Design review of the part shown in the three views and the two pictorial views. Dimensions are in mm from the part's minimum x, y and z. A direction names the side the tool comes from. Coordinates: 2 decimals unless noted, no trailing zeros. Loops run counter-clockwise (first coordinate to the right, second up) from the corner with the lowest first, then second, coordinate; pieces in that order, holes last. Notation, with made-up numbers: (-29.75, -25) -> (20.25, -25) arc R7 ccw to (20.25, -19) -> close; hole circle Ø9 at (16.25, 14.25). An arc over 180 degrees is marked (long way). Answer in a Markdown table with one row per item.
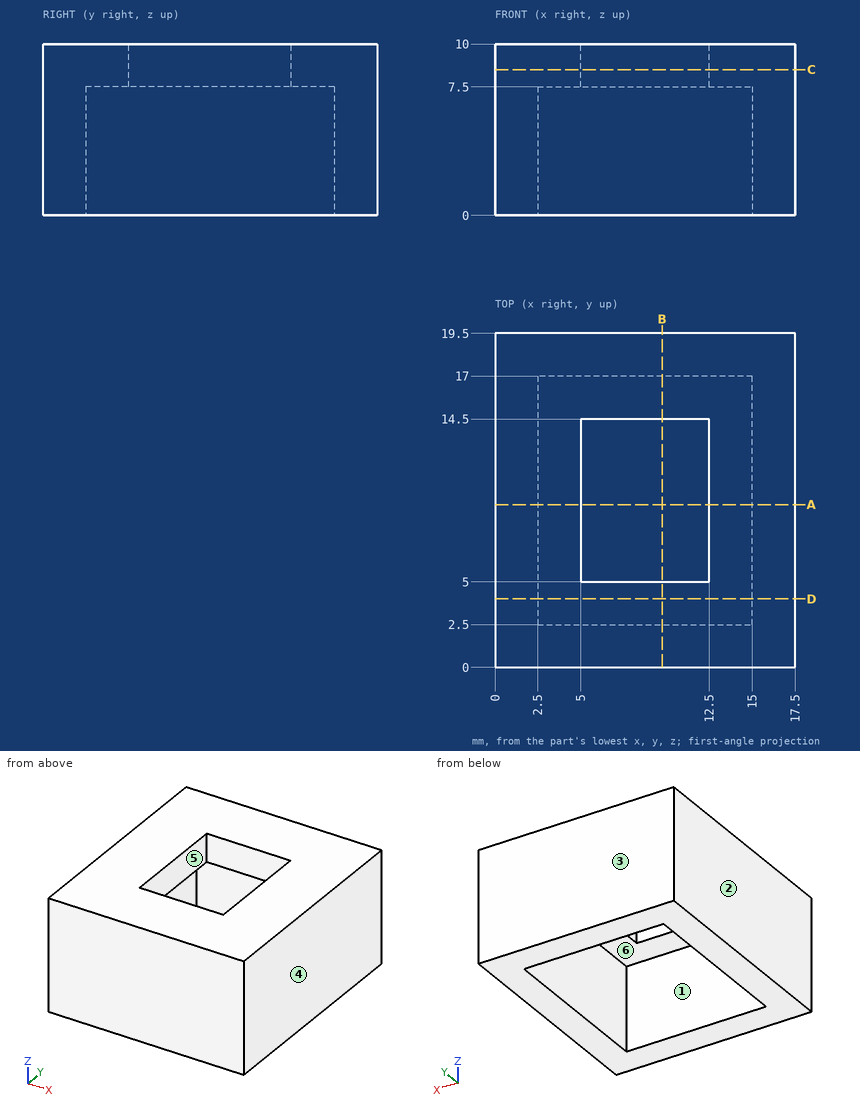
Item 1: Take a section at C-C, the plane z = 8.5. State the section outline as (x, y) points.
Worked answers:
| item | result |
|---|---|
| outline | (0, 0) -> (17.5, 0) -> (17.5, 19.5) -> (0, 19.5) -> close; hole (5, 5) -> (12.5, 5) -> (12.5, 14.5) -> (5, 14.5) -> close |
Item 2: For the marked faces 4, 5 and 6, list the 3-axis set-ups (+Z, -Z, +X, -X, +Y, -Y) from which the entire face can be reached by the end or side of a thin tool; tool diameter is ignored.
Worked answers:
| item | result |
|---|---|
| face 4 | +Z, -Z, +X, +Y, -Y |
| face 5 | +Z, -Z |
| face 6 | -Z |
Item 3: Take a section at A-A, the plane y = 9.5. State the section outline as (x, z) points.
Worked answers:
| item | result |
|---|---|
| outline | (0, 0) -> (2.5, 0) -> (2.5, 7.5) -> (5, 7.5) -> (5, 10) -> (0, 10) -> close; (12.5, 7.5) -> (15, 7.5) -> (15, 0) -> (17.5, 0) -> (17.5, 10) -> (12.5, 10) -> close |
Item 4: Insertion check: pin 1 (1.5 mm diameter, centred on y = 5.5, z = 8.5, fed in from -X); pin 2 (6 mm diameter, centred on x = 7, y = 11.5, fed in from -Z). Each pin has a flat end and moves straight along its axis. Give the tip position at first contact, or say it passes through.
Worked answers:
| item | result |
|---|---|
| pin 1 | x = 0 |
| pin 2 | z = 7.5 |
Item 5: The part is to be moulded in two halves that separate along Y. For the marked faces 1, 2 and 3, say which applies: +Y half, -Y half, draft (parallel to the pull), parting line (faces both ways), or undercut.
Worked answers:
| item | result |
|---|---|
| face 1 | undercut |
| face 2 | draft |
| face 3 | +Y half |
Item 6: For L1, parallel to Y at x = 11, z = 9.5; L2, parallel to X at y = 3, z = 0.5; L3, parallel to Y at x = 12.25, z = 4, list the stretches that pass through material, from the lowest coordinate up.
Worked answers:
| item | result |
|---|---|
| L1 | 0 to 5, 14.5 to 19.5 |
| L2 | 0 to 2.5, 15 to 17.5 |
| L3 | 0 to 2.5, 17 to 19.5 |
Item 7: Take a section at B-B, the plane x = 9.75. State the section outline as (y, z) points, and give its area (3 significant figures).
Worked answers:
| item | result |
|---|---|
| outline | (0, 0) -> (2.5, 0) -> (2.5, 7.5) -> (5, 7.5) -> (5, 10) -> (0, 10) -> close; (14.5, 7.5) -> (17, 7.5) -> (17, 0) -> (19.5, 0) -> (19.5, 10) -> (14.5, 10) -> close |
| area | 62.5 mm² |
Item 8: Take a section at D-D, the plane y = 4. State the section outline as (x, z) points.
Worked answers:
| item | result |
|---|---|
| outline | (0, 0) -> (2.5, 0) -> (2.5, 7.5) -> (15, 7.5) -> (15, 0) -> (17.5, 0) -> (17.5, 10) -> (0, 10) -> close |
